```python
from build123d import *

# Parameters (mm, degrees)
SKETCH004_R         = 4.175
PAD003_DEPTH        = 2
SKETCH005_R         = 3.175
PAD004_DEPTH        = 12.7
POCKET001_DEPTH     = 12.701
LINEARPATTERN_COUNT = 8
LINEARPATTERN_PITCH = 1.5


with BuildPart() as part:
    # Sketch004 → Pad003 (new body)
    with BuildSketch(Plane.XY):
        Circle(SKETCH004_R)
    extrude(amount=PAD003_DEPTH)

    # Sketch005 (on DatumPlane) → Pad004 (join)
    with BuildSketch(Plane.XY.offset(2)):
        Circle(SKETCH005_R)
    extrude(amount=PAD004_DEPTH)

    # Sketch006 (on DatumPlane) → Pocket001 (cut, through all)
    with BuildSketch(Plane.XY.offset(2)):
        Polygon((13.225, 0.525), (0.525, 0.525), (0.525, 13.225), (-0.525, 13.225), (-0.525, 0.525), (-13.225, 0.525), (-13.225, -0.525), (-0.525, -0.525), (-0.525, -13.225), (0.525, -13.225), (0.525, -0.525), (13.225, -0.525), align=None)
    extrude(amount=POCKET001_DEPTH, mode=Mode.SUBTRACT)

    # Sketch007 (on DatumPlane) → Groove (revolve, cut)
    with BuildSketch(Plane.XZ):
        Polygon((3.175, 14.7), (2.425, 13.95), (3.175, 13.2), align=None)
    groove = revolve(axis=Axis((0, 0, 0), (0, 0, 1)), mode=Mode.SUBTRACT)

    # LinearPattern: Groove ×8
    with Locations(*[(0, 0, -i * LINEARPATTERN_PITCH) for i in range(1, LINEARPATTERN_COUNT)]):
        add(groove, mode=Mode.SUBTRACT)


solid = part.part
```
Could you check a few things on this model? Use its own coordinates, in mm. A direction names the side the tool comes from. Round coordinates to 2 decimals unless told otherwise and drop trailing zeros. Write each loop counter-clockwise with the first axis right and the second up, starting at its lowest first coordinate (ties: lowest second). Pieces come first, ordered by that corner, then holes.
(1) Thinking about a two-plate mould opening in Z: for faces 1 (the face through (2, 0.525, 8)), 2 (the face through (1.94, 1.91, 6.15)), which applies, +Z half, -Z half, draft (parallel to the pull), parting line (faces both ways), or undercut?
Findings below:
face 1: draft
face 2: undercut
(2) Suppose I cut it at C-C on x = 0. Write out the boundary of the cut face in (y, z) (3 decimals), and give its area (3 significant figures).
Findings below:
outline: (-4.175, 0) - (4.175, 0) - (4.175, 2) - (-4.175, 2) - close
area: 16.7 mm2
(3) Which directions (+Z, -Z, +X, -X, +Y, -Y) give clear straight access to the entire face, cutting with the end or side of a thin tool? Please do faces 3 (the face through (-1.94, -1.91, 10.65)), 4 (the face through (1.94, 1.91, 3.15)), 5 (the face through (-1.901, 1.934, 5.236)).
Findings below:
face 3: -X, -Y
face 4: +X, +Y
face 5: -X, +Y
(4) Suppose I cut it at B-B on y = -2.75. State how many separate pieces and enclosed holes the cut face has, and give its area (3 significant figures).
Findings below:
separate pieces: 17
enclosed holes: 0
area: 21.4 mm2
(5) Suppose I cut it at A-A on z = 6. Write out the boundary of the cut face in (x, y) (3 decimals).
Findings below:
outline: (-2.827, -0.525) arc R2.875 ccw to (-0.525, -2.827) - (-0.525, -0.525) - close; (-2.827, 0.525) - (-0.525, 0.525) - (-0.525, 2.827) arc R2.875 ccw to start; (0.525, -2.827) arc R2.875 ccw to (2.827, -0.525) - (0.525, -0.525) - close; (0.525, 0.525) - (2.827, 0.525) arc R2.875 ccw to (0.525, 2.827) - close
(6) Suppose I cut it at D-D on z = 13.75. Write out the boundary of the cut face in (x, y) (3 decimals).
Findings below:
outline: (-2.572, -0.525) arc R2.625 ccw to (-0.525, -2.572) - (-0.525, -0.525) - close; (-2.572, 0.525) - (-0.525, 0.525) - (-0.525, 2.572) arc R2.625 ccw to start; (0.525, -2.572) arc R2.625 ccw to (2.572, -0.525) - (0.525, -0.525) - close; (0.525, 0.525) - (2.572, 0.525) arc R2.625 ccw to (0.525, 2.572) - close
(7) For pin 1 (2 mm diameter, centred on y = 2, z = 9, fed in from -X); pin 2 (5 mm diameter, centred on y = 2, z = 12, fed in from +X); pin 3 (5 mm diameter, centred on x = -1, z = 9, fed in from +Y), each with a flat end and sliding along its axis, tell me the tip position at first contact or that it passes through.
Findings below:
pin 1: stops at x = -3
pin 2: stops at x = 3.13
pin 3: stops at y = 3.13
(8) If I drill on probe 1 along Z at (x, y) = (3.25, 1.75); probe 2 along X at (y, z) = (-2, 12.75) (3 decimals); probe 3 along X at (y, z) = (1.25, 6.25) (3 decimals), over which ranges is the centre line in solid material (lowest first)?
Findings below:
probe 1: z = 0 to 2
probe 2: x = -1.851 to -0.525, 0.525 to 1.851
probe 3: x = -2.308 to -0.525, 0.525 to 2.308
